Input: part model. Units: mm. Frame: model coordinates. A direction names the side the tool comes from. Coordinates: 2 decimals unless noted, no trailing zeros. Loops run counter-clockwise (first coordinate to the right, second up) from the corner with the lowest first, then second, coordinate; pieces in that order, holes last.
(1) Section C-C, the plane z = 1. Return loops of the section in (x, y), then the cut area to 3 significant figures.
(2) Section D-D, the plane z = 2.5. Return loops of the section in (x, y).
(3) Line query: L1, parallel to Y at x = -2.25, z = -1.5; L2, parallel to X at y = 12.25, z = -1; L3, parallel to X at y = 8.5, z = -2.5. Output: solid intervals per line, ascending.
(4) Section B-B, the plane z = -0.5. Return loops of the section in (x, y).
(5) Set-up query: faces 1 (the face through (0, 0, 0)), 2 (the face through (0.423, 12.722, -1.763)). Return all of +Z, -Z, +X, -X, +Y, -Y with unobstructed straight access to the full face (end or side cutting, diameter ignored); none if empty.
(6) Mould query, pull axis X, two halves, no side actions, for faces 3 (the face through (0, 10, -0.25)), 4 (the face through (6.11, 4.82, -2.88)), 5 (the face through (-6.5, 5, 0)), 6 (the face through (0, 7, 3.25)). Classes: released by +X, released by -X, zero draft, split by the parting line, or undercut.
(7) Section A-A, the plane x = 0. Return loops of the section in (y, z).
(8) Contact query for flat-ended pins moving along their axis: P1, Ø1.5, axis at x = 4.5, y = 13.5, coming from the -Z side; P2, Ø1, axis at y = 10.5, z = 1.5, coming from the -X side; P3, Ø1.6, axis at x = 0, y = 8.5, coming from the -Z side. Output: stop coordinate, or through.
```python
from build123d import *

# Parameters (mm, degrees)
BASE_EXTRUDE_DEPTH = 3.25
SKETCH2_R          = 3.25
CUT_EXTRUDE1_DEPTH = 3
FILLET1_R          = 1.3
FILLET2_R          = 0.6


with BuildPart() as part:
    # Sketch1 → Base-Extrude (new, symmetric)
    with BuildSketch(Plane.XY):
        with BuildLine():
            Line((-6.5, 0), (6.5, 0))
            Line((6.5, 0), (6.5, 9.5))
            ThreePointArc((6.5, 9.5), (0, 16), (-6.5, 9.5))
            Line((-6.5, 9.5), (-6.5, 0))
        make_face()
    extrude(amount=BASE_EXTRUDE_DEPTH, both=True)

    # Sketch2 → Cut-Extrude1 (cut)
    with BuildSketch(Plane(origin=(0, 0, -3.25), x_dir=(-1, 0, 0), z_dir=(0, 0, -1))):
        with Locations((0, 9.5)):
            Circle(SKETCH2_R)
    extrude(amount=-CUT_EXTRUDE1_DEPTH, mode=Mode.SUBTRACT)

    # Fillet1
    fillet1_edges = [part.edges().sort_by_distance(p)[0] for p in [
        (6.5, 4.75, 3.25),
        (0, 16, 3.25),
        (-6.5, 4.75, 3.25),
        (0, 16, -3.25),
        (6.5, 4.75, -3.25),
        (-6.5, 4.75, -3.25),
    ]]
    fillet(fillet1_edges, radius=FILLET1_R)

    # Fillet2
    fillet2_edges = [part.edges().sort_by_distance(p)[0] for p in [
        (3.25, 9.5, -0.25),
        (3.25, 9.5, -3.25),
    ]]
    fillet(fillet2_edges, radius=FILLET2_R)


solid = part.part
```
Report:
1. outline: (-6.5, 0) - (6.5, 0) - (6.5, 9.5) arc R6.5 ccw to (-6.5, 9.5) - close
1. area: 190 mm2
2. outline: (-6.38, 0) - (6.38, 0) - (6.38, 9.5) arc R6.38 ccw to (-6.38, 9.5) - close
3. L1: y = 0 to 7.15, 11.85 to 15.6
3. L2: x = -5.89 to -1.73, 1.73 to 5.89
3. L3: x = -6.38 to -3.09, 3.09 to 6.38
4. outline: (-6.5, 0) - (6.5, 0) - (6.5, 9.5) arc R6.5 ccw to (-6.5, 9.5) - close; hole circle Ø6.27 at (0, 9.5)
5. face 1: +Z, -Z, +X, -X, -Y
5. face 2: -Z
6. face 3: undercut
6. face 4: released by +X
6. face 5: released by -X
6. face 6: zero draft
7. outline: (0, -3.25) - (5.65, -3.25) arc R0.6 ccw to (6.25, -2.65) - (6.25, -0.85) arc R0.6 cw to (6.85, -0.25) - (12.15, -0.25) arc R0.6 cw to (12.75, -0.85) - (12.75, -2.65) arc R0.6 ccw to (13.35, -3.25) - (14.7, -3.25) arc R1.3 ccw to (16, -1.95) - (16, 1.95) arc R1.3 ccw to (14.7, 3.25) - (0, 3.25) - close
8. P1: stops at z = -3.25
8. P2: stops at x = -6.48
8. P3: stops at z = -0.25
